Geometry: final body of the model. Coordinates: model frame, mm. A direction names the side the tool comes from. Round coordinates to 2 decimals unless told otherwise and drop trailing zeros. Write each loop counter-clockwise with the first axis right and the second up, starting at its lowest first coordinate (ties: lowest second). Pieces come first, ordered by that corner, then holes. Notation, with made-up numbers: M -38.5,61.5 L -0.5,61.5 A25 ccw -0.5,82.5 Z; hole C -16.5,88.25 d11. An arc over 180 degrees is marked long. Use one line per item in the form item = value. Start each with the question number.
Item 1: Pin query (flat end, axial travel): pin 1 Ø6 at (x, y) = (305, 59) entering from +Z; pin 2 Ø2 at (x, z) = (328, -50.5) entering from +Y. Return the tip coordinate at first contact, or that it passes through.
Item 2: Pull-direction query (Z, two-part tool) for faces 3 (the flat face through (182.41, 59.16, -8.984)), 4 (the flat face through (367, 62, -51)), 5 (the flat face through (184, 120, -19)); classes: pulls with the +Z half, pulls with the -Z half, needs draft (parallel to the pull), parting line crosses it, or undercut.
Item 3: Section query C-C (x = 239). Return loops of the section in (y, z), and give its area (3 significant figures).
Item 4: Section query D-D (y = 95). Return loops of the section in (x, z), and give its area (3 significant figures).
Item 5: Reachability of faces 1 (the flat face through (182.41, 60.84, -90.76)), 2 (the flat face through (182.452, 62.319, -87.502)) from +Z, -Z, +X, -X, +Y, -Y: full face, straight path, thin tool, end or side. Return the list, or none.
Item 6: Section query A-A (z = -39.5). Return loops of the section in (x, y), and give its area (3 significant figures).
Item 7: Ray query, probe 1 along X at (y, z) = (66.5, -16.5); probe 2 along Z at (x, y) = (146, 21); probe 3 along Z at (x, y) = (113, 33). Return the intervals inside material, ascending.
Item 8: Section query B-B (y = 20.5). Return loops of the section in (x, z).
from build123d import *

# Parameters (mm, degrees)
BOSS_EXTRUDE1_DEPTH = 370
SHELL1_T            = -3
BOSS_EXTRUDE2_REACH = 398.278
SKETCH3_W           = 50
SKETCH3_H           = 3


with BuildPart() as part:
    # Sketch2 → Boss-Extrude1 (new body)
    with BuildSketch(Plane(origin=(0, 0, 0), x_dir=(0, 0, -1), z_dir=(1, 0, 0))):
        Polygon((100, 0), (0, 0), (18.222222222, 120), (81.777777778, 120), align=None)
    extrude(amount=BOSS_EXTRUDE1_DEPTH)

    # Shell1
    shell1_openings = [part.faces().sort_by_distance(p)[0] for p in [
        (185, 120, -50),
    ]]
    offset(amount=SHELL1_T, openings=shell1_openings, kind=Kind.INTERSECTION)

    # Boss-Extrude2: up to this plane
    boss_extrude2_end = Plane(origin=(370, 119.549607645, -21.188220659), z_dir=(0, -0.15013078506635866, -0.9886661455594395))
    # Sketch3 → Boss-Extrude2 (add, up to the surface)
    with BuildSketch(Plane(origin=(0, 14.392530105, -94.780076301), x_dir=(1, 0, 0), z_dir=(0, -0.1501307850664947, 0.988666145559419)), mode=Mode.PRIVATE) as boss_extrude2_sk1:
        with Locations((305, 29.976868399)):
            Rectangle(SKETCH3_W, SKETCH3_H)
    boss_extrude2_tool1 = split(extrude(boss_extrude2_sk1.sketch, amount=BOSS_EXTRUDE2_REACH, mode=Mode.PRIVATE), bisect_by=boss_extrude2_end, keep=Keep.BOTH, mode=Mode.PRIVATE)
    add(boss_extrude2_tool1.solids().sort_by_distance((305, 44.029645, -90.279626))[0])


solid = part.part
Working result:
q1.pin_1 = -8.5
q1.pin_2 = 39.66
q2.face_3 = pulls with the +Z half
q2.face_4 = undercut
q2.face_5 = needs draft
q3.outline = M 0,-100 L 120,-81.78 L 120,-78.74 L 3,-96.51 L 3,-3.49 L 120,-21.26 L 120,-18.22 L 0,0 Z
q3.area = 1,010 mm²
q4.outline = M 0,-85.57 L 370,-85.57 L 370,-14.43 L 0,-14.43 Z; hole M 3,-82.54 L 367,-82.54 L 367,-17.46 L 3,-17.46 Z
q4.area = 2,640 mm²
q5.face_1 = -Z, +X, -X, +Y
q5.face_2 = none
q6.outline = M 0,0 L 370,0 L 370,120 L 367,120 L 367,3 L 3,3 L 3,120 L 0,120 Z; M 280,34.8 L 330,34.8 L 330,37.84 L 280,37.84 Z
q6.area = 1,960 mm²
q7.probe_1 = 0 to 3, 367 to 370
q7.probe_2 = -96.81 to -93.78, -6.22 to -3.19
q7.probe_3 = -94.99 to -91.95, -8.05 to -5.01
q8.outline = M 0,-96.89 L 370,-96.89 L 370,-3.11 L 0,-3.11 Z; hole M 3,-93.85 L 367,-93.85 L 367,-6.15 L 3,-6.15 Z
